Study the drawing (mm; zero at the part's minimum x, y, z) and answer. A direction names the side the tool comes from. Coordinates: 2 decimals unless noted, no trailing zeros. Loops run counter-clockwise (first coordinate to the right, second up) from the corner with the lowest first, then second, coordinate; pieces in that order, holes last. Notation, with made-up numbers: (26, 67.5) -> (42, 67.5) arc R26 ccw to (42, 93.5) -> close; hole circle Ø7 at (-25.75, -28.5). An arc over 180 degrees is marked (long way). Answer as CSV lines item,"result".
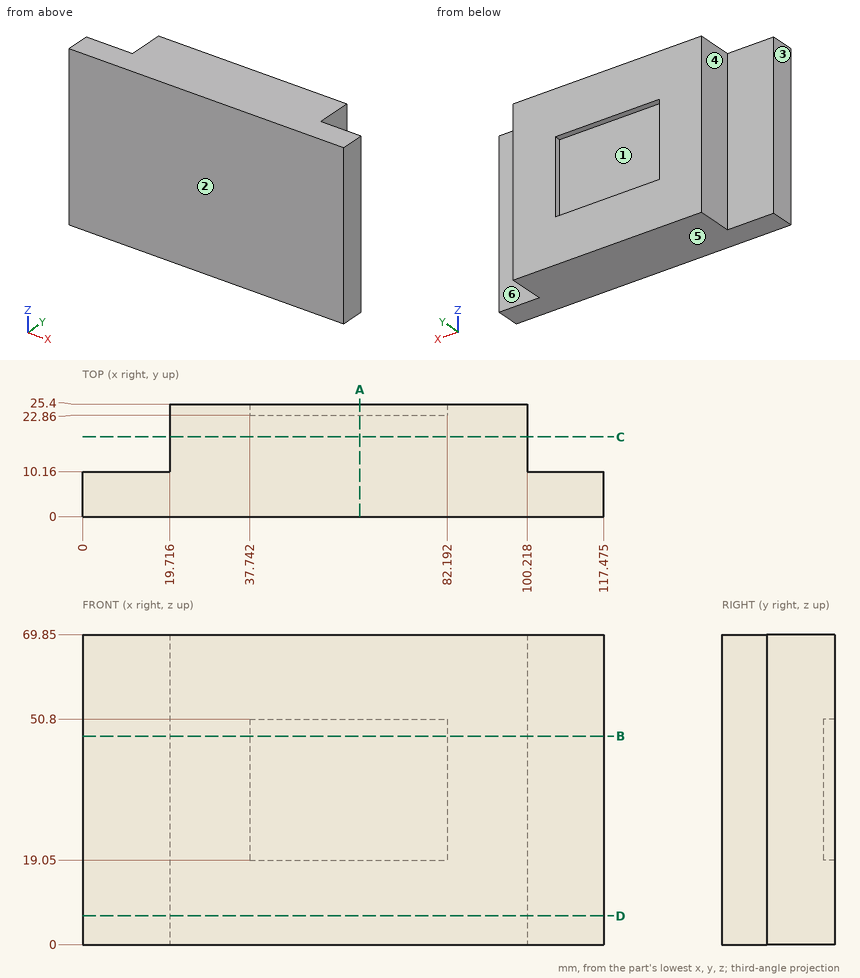
Q1. A cutting plane is placed at B-B, the plane z = 47. Write down the section's boundary in (x, y) (1 decimal).
Results:
outline,"(0, 0) -> (117.5, 0) -> (117.5, 10.2) -> (100.2, 10.2) -> (100.2, 25.4) -> (82.2, 25.4) -> (82.2, 22.9) -> (37.7, 22.9) -> (37.7, 25.4) -> (19.7, 25.4) -> (19.7, 10.2) -> (0, 10.2) -> close"
Q2. For a pull along X with two mould halves and no side action, classify the marked faces 1, 2 and 3 as pulls with the +X half, pulls with the -X half, needs draft (parallel to the pull), parting line crosses it, or undercut.
Results:
face 1,"undercut"
face 2,"needs draft"
face 3,"pulls with the -X half"
Q3. Given pin 1 Ø12 at (y, z) = (18.5, 20.5) entering from -X; pin 2 Ø6 at (y, z) = (15.5, 18.5) entering from +X; pin 3 Ø8.5 at (x, z) = (113, 18.5) entering from +Y, each flat-ended and moving along its own axis, determine where each tip first touches the part or whether it passes through.
Results:
pin 1,"stops at x = 19.72"
pin 2,"stops at x = 100.22"
pin 3,"stops at y = 10.16"
Q4. A cutting plane is placed at A-A, the plane x = 62.5. Write down the section's boundary in (y, z), and give its area (3 significant figures).
Results:
outline,"(0, 0) -> (25.4, 0) -> (25.4, 19.05) -> (22.86, 19.05) -> (22.86, 50.8) -> (25.4, 50.8) -> (25.4, 69.85) -> (0, 69.85) -> close"
area,"1,690 mm²"
Q5. A cutting plane is placed at C-C, the plane y = 18. Write down the section's boundary in (x, z), and give its area (3 significant figures).
Results:
outline,"(19.72, 0) -> (100.22, 0) -> (100.22, 69.85) -> (19.72, 69.85) -> close"
area,"5,620 mm²"
Q6. A cutting plane is placed at D-D, the plane z = 6.5. Write down the section's boundary in (x, y) (1 decimal), and give its area (3 significant figures).
Results:
outline,"(0, 0) -> (117.5, 0) -> (117.5, 10.2) -> (100.2, 10.2) -> (100.2, 25.4) -> (19.7, 25.4) -> (19.7, 10.2) -> (0, 10.2) -> close"
area,"2,420 mm²"
Q7. Find the intervals of material crossed by probe 1 along Z at (x, y) = (66.5, 23.75); probe 2 along Y at (x, z) = (101, 14.5); probe 3 along Y at (x, z) = (70, 30), in increasing order. Write a range as [from, to].
Results:
probe 1,"z = [0, 19.05], [50.8, 69.85]"
probe 2,"y = [0, 10.16]"
probe 3,"y = [0, 22.86]"
Q8. For the marked faces 4, 5 and 6, determine the directions among +Z, -Z, +X, -X, +Y, -Y from which every point of the face is accessible in a straight line to the end or side of a thin tool.
Results:
face 4,"+Z, -Z, -X, +Y"
face 5,"-Z, +X, -X, +Y, -Y"
face 6,"+Z, -Z, +X, +Y"
